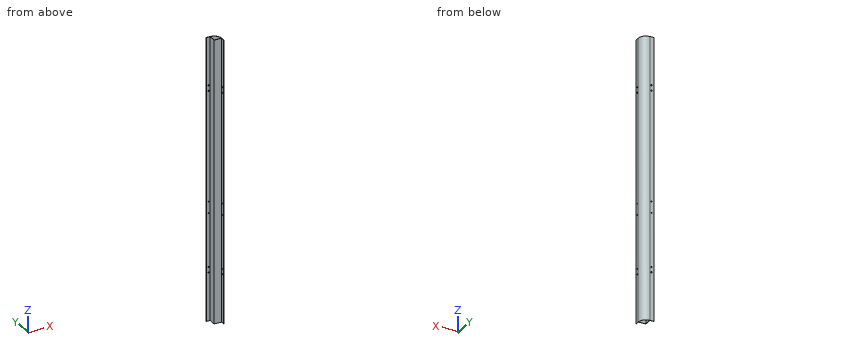
```python
from build123d import *

# Parameters (mm, degrees)
CROQUIS1_W              = 13
CROQUIS1_H              = 1
CROQUIS1_W_2            = 1
CROQUIS1_H_2            = 13
SALIENTE_EXTRUIR1_DEPTH = 500
CROQUIS2_R              = 2.38125
CROQUIS2_R_2            = 1.5
CORTAR_EXTRUIR1_DEPTH   = 10
CROQUIS3_R              = 2.38125
CROQUIS3_R_2            = 1.5
CORTAR_EXTRUIR2_DEPTH   = 10


with BuildPart() as part:
    # Croquis1 → Saliente-Extruir1 (new body, symmetric)
    with BuildSketch(Plane.XY):
        with BuildLine():
            ThreePointArc((-13.7, 13.681053808), (5.967619023, 5.967619023), (13.681053808, -13.7))
            Line((13.681053808, -13.7), (-13.7, -13.7))
            Line((-13.7, -13.7), (-13.7, 13.681053808))
        make_face()
        with BuildLine():
            Line((-12.7, -12.7), (-12.7, 12.7))
            ThreePointArc((-12.7, 12.7), (5.260512242, 5.260512242), (12.7, -12.7))
            Line((12.7, -12.7), (-12.7, -12.7))
        make_face(mode=Mode.SUBTRACT)
        with Locations((-20.2, 13.181053808)):
            Rectangle(CROQUIS1_W, CROQUIS1_H)
        with Locations((13.181053808, -20.2)):
            Rectangle(CROQUIS1_W_2, CROQUIS1_H_2)
    extrude(amount=SALIENTE_EXTRUIR1_DEPTH, both=True)

    # Croquis2 → Cortar-Extruir1 (cut)
    with BuildSketch(Plane(origin=(13.681053808, 0, 0), x_dir=(0, 0, -1), z_dir=(1, 0, 0))):
        with Locations((310.5, -18.7)):
            Circle(CROQUIS2_R)
        with Locations((329.5, -18.7)):
            Circle(CROQUIS2_R)
        with Locations((-329.5, -18.7)):
            Circle(CROQUIS2_R)
        with Locations((-310.5, -18.7)):
            Circle(CROQUIS2_R)
        with Locations((120, -18.7)):
            Circle(CROQUIS2_R_2)
        with Locations((80, -18.7)):
            Circle(CROQUIS2_R_2)
    extrude(amount=-CORTAR_EXTRUIR1_DEPTH, mode=Mode.SUBTRACT)

    # Croquis3 → Cortar-Extruir2 (cut)
    with BuildSketch(Plane(origin=(0, 13.681053808, 0), x_dir=(1, 0, 0), z_dir=(0, 1, 0))):
        with Locations((-18.7, 329.5)):
            Circle(CROQUIS3_R)
        with Locations((-18.7, 310.5)):
            Circle(CROQUIS3_R)
        with Locations((-18.7, -310.5)):
            Circle(CROQUIS3_R)
        with Locations((-18.7, -329.5)):
            Circle(CROQUIS3_R)
        with Locations((-18.7, 120)):
            Circle(CROQUIS3_R_2)
        with Locations((-18.7, 80)):
            Circle(CROQUIS3_R_2)
    extrude(amount=-CORTAR_EXTRUIR2_DEPTH, mode=Mode.SUBTRACT)


solid = part.part
```
The listing builds one solid part. Answer for the finished solid, in the listing's coordinates (mm). Give positions to 0.01 mm unless a question says otherwise; leave off trailing zeros. Order: outer loops, then holes, each group sorted by start corner. A loop starts at its lowest first (then second) coordinate and runs counter-clockwise, first axis right, second up. Notation, with made-up numbers: (-23.5, -7) - (16.5, -7) arc R19 ccw to (16.5, 13) - close; hole circle Ø10 at (-2.5, -25.75). An arc over 180 degrees is marked (long way). Answer in a Markdown table with one row per item. Add a question column.
Q1. Find the intervals of material crossed by line 1 along X through (y, z) = (-21, 107); line 2 along Y through (x, z) = (10, -348), in increasing order. Write a range as [from, to].
Q2. The part is cut by section B-B (z = 5). Determine the outline of the cut face in (x, y), then the cut area to 3 significant figures.
Q3. The part is cut by section C-C (y = 2). Determine the outline of the cut face in (x, z).
Q4. The part is cut by section A-A (x = -3). Determine the outline of the cut face in (y, z), then the cut area to 3 significant figures.
Q5. Given P1, Ø5.5, axis at y = -18.7, z = 310.5, coming from the +X side; P2, Ø7.5, axis at y = -18.7, z = -310.5, coming from the -X side; P3, Ø5, axis at y = -11, z = -198, coming from the -X side; P4, Ø5, axis at x = -17, y = -15.5, coming from the -Z side, each flat-ended and moving along its own axis, determine where each tip first touches the part or whether it passes through.
Determined:
| question | item | result |
|---|---|---|
| 1 | line 1 | x = [12.68, 13.68] |
| 1 | line 2 | y = [-13.7, -12.7], [-1.3, 0.78] |
| 2 | outline | (-26.7, 12.68) - (-13.7, 12.68) - (-13.7, -13.7) - (12.68, -13.7) - (12.68, -26.7) - (13.68, -26.7) - (13.68, -13.7) arc R26.4 ccw to (-13.7, 13.68) - (-26.7, 13.68) - close; hole (-12.7, -12.7) - (12.7, -12.7) arc R25.4 ccw to (-12.7, 12.7) - close |
| 2 | area | 120 mm² |
| 3 | outline | (-13.7, -500) - (-12.7, -500) - (-12.7, 500) - (-13.7, 500) - close; (8.01, -500) - (9.23, -500) - (9.23, 500) - (8.01, 500) - close |
| 4 | outline | (-13.7, -500) - (-12.7, -500) - (-12.7, 500) - (-13.7, 500) - close; (10.77, -500) - (11.85, -500) - (11.85, 500) - (10.77, 500) - close |
| 4 | area | 2,080 mm² |
| 5 | P1 | stops at x = 13.68 |
| 5 | P2 | stops at x = 12.68 |
| 5 | P3 | stops at x = -13.7 |
| 5 | P4 | passes through |
